Geometry: final body of the model. Coordinates: model frame, mm. Face numbers are marked on the shaded views. A direction names the side the tool comes from. Give positions to 0.01 mm unless a question says otherwise; leave off trailing zeros. Write each loop counter-clockwise with the first axis right and the second up, starting at its lowest first coordinate (ties: lowest second). Pieces come first, ordered by that corner, then holes.
from build123d import *

# Parameters (mm, degrees)
EXTRUDE_1_DEPTH          = 15
SKETCH_2_R               = 5.15
CUT_EXTRUDE_1_DEPTH      = 15
EXTRUDE_3_DEPTH          = 15
SKETCH_5_W               = 5
SKETCH_5_H               = 10
CUT_EXTRUDE_3_DEPTH      = 15
CUT_EXTRUDE_4_DEPTH      = 15
CUT_EXTRUDE_4_DEPTH_BACK = 27
SKETCH_6_R               = 3.25
SKETCH_7_R               = 1.5
CUT_EXTRUDE_5_DEPTH      = 3.5
CUT_EXTRUDE_7_DEPTH      = 15
EXTRUDE_4_REACH          = 135.688
SKETCH_12_R              = 1.75
CUT_EXTRUDE_9_DEPTH      = 50
CUT_EXTRUDE_10_DEPTH     = 3
SKETCH_14_R              = 1.65
CUT_EXTRUDE_11_DEPTH     = 5
SKETCH_15_R              = 5.15
CUT_EXTRUDE_12_DEPTH     = 15
CUT_EXTRUDE_13_DEPTH     = 15
CUT_EXTRUDE_14_DEPTH     = 15
SKETCH_18_W              = 30
SKETCH_18_H              = 15
CUT_EXTRUDE_15_DEPTH     = 15
CUT_EXTRUDE_16_DEPTH     = 135
FILLET_3_R               = 10
FILLET_4_R               = 2
FILLET_5_R               = 5
EXTRUDE_5_DEPTH          = 5
FILLET_6_R               = 1
CUT_EXTRUDE_17_DEPTH     = 0.5
SKETCH_22_R              = 1.65
EXTRUDE_6_DEPTH          = 0.5
SCALE_1_SCALE            = 0.6


with BuildPart() as part:
    # 草图1 → 凸台-拉伸1 (new body)
    with BuildSketch(Plane.XY):
        with BuildLine():
            Line((40, 7.5), (-40, 7.5))
            Line((-40, 7.5), (-40, -7.5))
            Line((-40, -7.5), (39.456922296, -7.5))
            add(Edge.make_bspline(
                [(39.456922296, -7.5), (46.411815441, -13.348879485), (59.483442953, -20.788944656), (71.646457346, -24.94425278), (84, -26.35191574), (96.353542654, -24.94425278), (108.516557047, -20.788944656), (123.382931224, -12.327351589), (132.036036764, -4.43964044)],
                knots=[0.037726639, 0.037726639, 0.037726639, 0.1875, 0.3125, 0.4375, 0.5625, 0.6875, 0.8125, 1, 1, 1], degree=2))
            Line((132.036036764, -4.43964044), (123.963963236, 4.43964044))
            add(Edge.make_bspline(
                [(44.036036764, 4.43964044), (51.882931224, -2.672648411), (64.516557047, -9.836055344), (74.353542654, -13.18074722), (84, -14.27308426), (93.646457346, -13.18074722), (103.483442953, -9.836055344), (116.117068776, -2.672648411), (123.963963236, 4.43964044)],
                knots=[0, 0, 0, 0.1875, 0.3125, 0.4375, 0.5625, 0.6875, 0.8125, 1, 1, 1], degree=2))
            Line((44.036036764, 4.43964044), (40, 7.5))
        make_face()
    extrude(amount=EXTRUDE_1_DEPTH)

    # 草图2 → 切除-拉伸1 (cut)
    with BuildSketch(Plane(origin=(0, 7.5, 0), x_dir=(1, 0, 0), z_dir=(0, 1, 0))):
        with Locations(Location((0, -7.5, 0), (0, 0, 270))):
            Circle(SKETCH_2_R)
    extrude(amount=-CUT_EXTRUDE_1_DEPTH, mode=Mode.SUBTRACT)

    # 草图4 → 凸台-拉伸3 (add)
    with BuildSketch(Plane(origin=(0, 0, 0), x_dir=(-1, 0, 0), z_dir=(0, 0, -1))):
        Polygon((-40, 7.5), (-44.036036764, 7.5), (-44.036036764, 4.43964044), align=None)
    extrude(amount=-EXTRUDE_3_DEPTH)

    # 草图5 → 切除-拉伸3 (cut)
    with BuildSketch(Plane(origin=(0, 0, 0), x_dir=(-1, 0, 0), z_dir=(0, 0, -1))):
        with Locations((-11.65, 2.5)):
            Rectangle(SKETCH_5_W, SKETCH_5_H)
    extrude(amount=-CUT_EXTRUDE_3_DEPTH, mode=Mode.SUBTRACT)

    # 草图6 → 切除-拉伸4 (cut, two sides: drawn at the far end of the back side and taken through both)
    with BuildSketch(Plane(origin=(44.036036764, 0, 0), x_dir=(0, 0, -1), z_dir=(1, 0, 0)).offset(-CUT_EXTRUDE_4_DEPTH_BACK)):
        with Locations(Location((-7.5, 2.5, 0), (0, 0, 143.358054803))):
            Circle(SKETCH_6_R)
    extrude(amount=CUT_EXTRUDE_4_DEPTH + CUT_EXTRUDE_4_DEPTH_BACK, mode=Mode.SUBTRACT)

    # 草图7 → 切除-拉伸5 (cut)
    with BuildSketch(Plane(origin=(9.15, 0, 0), x_dir=(0, 0, -1), z_dir=(1, 0, 0))):
        with Locations((-7.5, 2.5)):
            Circle(SKETCH_7_R)
    extrude(amount=-CUT_EXTRUDE_5_DEPTH, mode=Mode.SUBTRACT)

    # 草图9 → 切除-拉伸7 (cut)
    with BuildSketch(Plane(origin=(0, 0, 0), x_dir=(-1, 0, 0), z_dir=(0, 0, -1))):
        with BuildLine():
            Line((-49, -14.628935139), (-119, -14.628935139))
            add(Edge.make_bspline(
                [(-49, -14.628935139), (-51.259755236, -16.108213622), (-59.483442953, -20.788944656), (-71.646457346, -24.94425278), (-84, -26.35191574), (-96.353542654, -24.94425278), (-108.516557047, -20.788944656), (-116.740244764, -16.108213622), (-119, -14.628935139)],
                knots=[0.139633208, 0.139633208, 0.139633208, 0.1875, 0.3125, 0.4375, 0.5625, 0.6875, 0.8125, 0.860366792, 0.860366792, 0.860366792], degree=2))
        make_face()
    extrude(amount=-CUT_EXTRUDE_7_DEPTH, mode=Mode.SUBTRACT)

    # 凸台-拉伸4: up to this face of the body (flat: up to its plane)
    extrude_4_end = Plane(part.part.faces().sort_by_distance((30.242148565, -2.823725013, 15))[0])
    # 草图10 → 凸台-拉伸4 (add, up to the picked face)
    with BuildSketch(Plane(origin=(0, 0, 0), x_dir=(-1, 0, 0), z_dir=(0, 0, -1)), mode=Mode.PRIVATE) as extrude_4_sk1:
        with BuildLine():
            Line((-114, -3.531559291), (-54, -3.531559291))
            add(Edge.make_bspline(
                [(-54, -3.531559291), (-56.748654683, -5.431567952), (-64.516557047, -9.836055344), (-74.353542654, -13.18074722), (-84, -14.27308426), (-93.646457346, -13.18074722), (-103.483442953, -9.836055344), (-111.251345317, -5.431567952), (-114, -3.531559291)],
                knots=[0.120356468, 0.120356468, 0.120356468, 0.1875, 0.3125, 0.4375, 0.5625, 0.6875, 0.8125, 0.879643532, 0.879643532, 0.879643532], degree=2))
        make_face()
    extrude_4_tool1 = split(extrude(extrude_4_sk1.sketch, amount=-EXTRUDE_4_REACH, mode=Mode.PRIVATE), bisect_by=extrude_4_end, keep=Keep.BOTH, mode=Mode.PRIVATE)
    add(extrude_4_tool1.solids().sort_by(Axis((84, -7.71433, 0), (0, 0, 1)))[0])

    # 草图12 → 切除-拉伸9 (cut)
    with BuildSketch(Plane(origin=(0, -3.531559291, 0), x_dir=(1, 0, 0), z_dir=(0, 1, 0))):
        with Locations(Location((74.000000001, -7.5, 0), (0, 0, 180))):
            Circle(SKETCH_12_R)
        with Locations(Location((104.000000001, -7.5, 0), (0, 0, 180))):
            Circle(SKETCH_12_R)
    extrude(amount=-CUT_EXTRUDE_9_DEPTH, mode=Mode.SUBTRACT)

    # 草图13 → 切除-拉伸10 (cut)
    with BuildSketch(Plane.XZ.offset(14.628935139)):
        Polygon((75.674315782, 4.6), (77.348631563, 7.5), (75.674315782, 10.4), (72.325684221, 10.4), (70.65136844, 7.5), (72.325684221, 4.6), align=None)
        Polygon((105.674315782, 4.6), (107.348631563, 7.5), (105.674315782, 10.4), (102.325684221, 10.4), (100.65136844, 7.5), (102.325684221, 4.6), align=None)
    extrude(amount=-CUT_EXTRUDE_10_DEPTH, mode=Mode.SUBTRACT)

    # 草图14 → 切除-拉伸11 (cut)
    with BuildSketch(Plane(origin=(17.036036764, 0, 0), x_dir=(0, 0, -1), z_dir=(1, 0, 0))):
        with Locations((-7.5, 2.5)):
            Circle(SKETCH_14_R)
    extrude(amount=-CUT_EXTRUDE_11_DEPTH, mode=Mode.SUBTRACT)

    # 草图15 → 切除-拉伸12 (cut)
    with BuildSketch(Plane(origin=(0, 7.5, 0), x_dir=(1, 0, 0), z_dir=(0, 1, 0))):
        with Locations(Location((26.05, -7.5, 0), (0, 0, 270))):
            Circle(SKETCH_15_R)
    extrude(amount=-CUT_EXTRUDE_12_DEPTH, mode=Mode.SUBTRACT)

    # 草图16 → 切除-拉伸13 (cut)
    with BuildSketch(Plane(origin=(0, 0, 0), x_dir=(-1, 0, 0), z_dir=(0, 0, -1))):
        Polygon((-44.036036764, 4.43964044), (-40.036036764, 7.5), (-44.036036764, 7.5), align=None)
    extrude(amount=-CUT_EXTRUDE_13_DEPTH, mode=Mode.SUBTRACT)

    # 草图17 → 切除-拉伸14 (cut)
    with BuildSketch(Plane(origin=(0, 0, 0), x_dir=(-1, 0, 0), z_dir=(0, 0, -1))):
        Polygon((-114, -3.531559291), (-155.45087664, -3.531559291), (-96.986746886, 29.708253825), align=None)
    extrude(amount=-CUT_EXTRUDE_14_DEPTH, mode=Mode.SUBTRACT)

    # 草图18 → 切除-拉伸15 (cut)
    with BuildSketch(Plane(origin=(0, 0, 0), x_dir=(-1, 0, 0), z_dir=(0, 0, -1))):
        with Locations((25, 0)):
            Rectangle(SKETCH_18_W, SKETCH_18_H)
    extrude(amount=-CUT_EXTRUDE_15_DEPTH, mode=Mode.SUBTRACT)

    # 草图19 → 切除-拉伸16 (cut)
    with BuildSketch(Plane.XY.offset(15)):
        Polygon((119, -14.628935139), (127.815134708, -3.531559292), (136.052125617, -3.531559292), align=None)
    extrude(amount=-CUT_EXTRUDE_16_DEPTH, mode=Mode.SUBTRACT)

    # 圆角3
    fillet_3_edges = [part.edges().sort_by_distance(p)[0] for p in [
        (119, -14.628935139, 7.5),
    ]]
    fillet(fillet_3_edges, radius=FILLET_3_R)

    # 圆角4
    fillet_4_edges = [part.edges().sort_by_distance(p)[0] for p in [
        (127.815134708, -3.531559292, 7.5),
    ]]
    fillet(fillet_4_edges, radius=FILLET_4_R)

    # 圆角5
    fillet_5_edges = [part.edges().sort_by_distance(p)[0] for p in [
        (-10, 0, 15),
        (-10, 0, 0),
    ]]
    fillet(fillet_5_edges, radius=FILLET_5_R)

    # 草图20 → 凸台-拉伸5 (add)
    with BuildSketch(Plane(origin=(9.15, 0, 0), x_dir=(0, 0, -1), z_dir=(1, 0, 0))):
        Polygon((-10, -2.5), (-15, -2.5), (-15, 5.5), align=None)
        Polygon((0, 5.5), (-5, -2.5), (0, -2.5), align=None)
    extrude(amount=EXTRUDE_5_DEPTH)

    # 圆角6
    fillet_6_edges = [part.edges().sort_by_distance(p)[0] for p in [
        (11.65, 5.5, 15),
        (11.65, 5.5, 0),
    ]]
    fillet(fillet_6_edges, radius=FILLET_6_R)

    # 草图21 → 切除-拉伸17 (cut)
    with BuildSketch(Plane(origin=(9.15, 0, 0), x_dir=(0, 0, -1), z_dir=(1, 0, 0))):
        with BuildLine():
            Line((-5, -2.5), (-1.847998304, 2.543202714))
            ThreePointArc((-1.847998304, 2.543202714), (-0.724317487, 2.97445252), (0, 2.013203774))
            Line((0, 2.013203774), (0, 7.5))
            Line((0, 7.5), (-15, 7.5))
            Line((-15, 7.5), (-15, 2.013203774))
            ThreePointArc((-15, 2.013203774), (-14.275682513, 2.97445252), (-13.152001696, 2.543202714))
            Line((-13.152001696, 2.543202714), (-10, -2.5))
            Line((-10, -2.5), (-5, -2.5))
        make_face()
    extrude(amount=-CUT_EXTRUDE_17_DEPTH, mode=Mode.SUBTRACT)

    # 草图22 → 凸台-拉伸6 (add)
    with BuildSketch(Plane.ZY.offset(-14.15)):
        with BuildLine():
            Line((0, 7.5), (0, 2.013203774))
            ThreePointArc((0, 2.013203774), (0.724317487, 2.97445252), (1.847998304, 2.543202714))
            Line((1.847998304, 2.543202714), (5, -2.5))
            Line((5, -2.5), (10, -2.5))
            Line((10, -2.5), (13.152001696, 2.543202714))
            ThreePointArc((13.152001696, 2.543202714), (14.275682513, 2.97445252), (15, 2.013203774))
            Line((15, 2.013203774), (15, 7.5))
            Line((15, 7.5), (0, 7.5))
        make_face()
        with Locations(Location((7.5, 2.5, 0), (0, 0, 180))):
            Circle(SKETCH_22_R, mode=Mode.SUBTRACT)
    extrude(amount=EXTRUDE_6_DEPTH)


with BuildPart() as part_1:
    # 缩放比例1: scaled about (0, 0, 0)
    add(part.part.scale(SCALE_1_SCALE))


solid = part_1.part
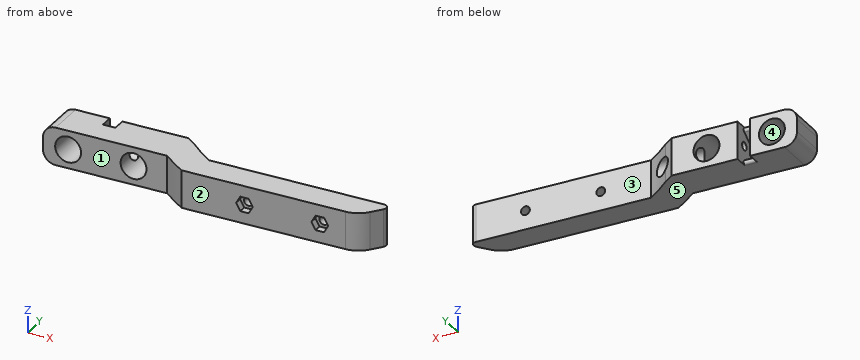
Q1. Section C-C on x = 15.63. Output: boundary loops of the cut face in (y, z).
Filled sheet:
outline: (-4.5, 0) - (4.5, 0) - (4.5, 1.41) - (-4.5, 1.41) - close; (-4.5, 7.59) - (4.5, 7.59) - (4.5, 9) - (-4.5, 9) - close
Q2. Pull-direction query (Z, two-part tool) for the marked faces 3, 4 and 5; classes: released by +Z, released by -Z, zero draft, split by the parting line, or undercut.
Filled sheet:
face 3: zero draft
face 4: undercut
face 5: released by -Z
Q3. Ray query, line 1 along Z through (x, y) = (62.4, -3.75); line 2 along X through (y, z) = (-1.75, 6); line 3 along X through (y, z) = (2.25, 5.75). Return the intervals inside material, ascending.
Filled sheet:
line 1: z = 0 to 3.45, 5.55 to 9
line 2: x = -6 to -2.7, 2.7 to 12.93, 18.33 to 31.87
line 3: x = -6 to -2.83, 2.83 to 5.19, 8.19 to 10.22
Q4. Section B-B on y = -3.25. Output: boundary loops of the cut face in (x, z), plus the area to 3 significant figures.
Filled sheet:
outline: (-6, 3) arc R3 ccw to (-3, 0) - (75.4, 0) - (75.4, 9) - (-3, 9) arc R3 ccw to (-6, 6) - close; hole circle Ø6.18 at (0, 4.5); hole circle Ø6.18 at (15.63, 4.5); hole circle Ø2.1 at (44.4, 4.5); hole circle Ø2.1 at (62.4, 4.5)
area: 662 mm2
Q5. Pin query (flat end, axial travel): P1, Ø4.5, axis at y = 1.5, z = 4.5, coming from the +X side; P2, Ø0.9, axis at x = 63, y = -7.5, coming from the -Z side; P3, Ø1.7, axis at x = 62.4, z = 4.5, coming from the -Y side; P4, Ø0.9, axis at x = 6.5, z = 4, coming from the +Y side. Return the tip coordinate at first contact, or that it passes through.
Filled sheet:
P1: stops at x = 30.51
P2: stops at z = 0
P3: passes through
P4: stops at y = -1.5
Q6. Access query for the marked faces 1 and 2. Directions: +Z, -Z, +X, -X, +Y, -Y. A direction counts if a zero-diameter tool reaches every point of the face in a straight line with its end or side. Return the directions, or none.
Filled sheet:
face 1: +Z, -Z, -X, -Y
face 2: +Z, -Z, +X, -X, -Y
Q7. Section D-D on x = 55. Output: boundary loops of the cut face in (y, z), plus the area to 3 significant figures.
Filled sheet:
outline: (-8.78, 0) - (-2.12, 0) - (-2.12, 9) - (-8.78, 9) - close
area: 59.9 mm2
Q8. Section A-A on x = 44.4. Output: boundary loops of the cut face in (y, z), plus the area to 3 significant figures.
Filled sheet:
outline: (-8.78, 0) - (-2.12, 0) - (-2.12, 3.45) - (-6.98, 3.45) - (-6.98, 2.76) - (-8.78, 2.76) - close; (-8.78, 6.24) - (-6.98, 6.24) - (-6.98, 5.55) - (-2.12, 5.55) - (-2.12, 9) - (-8.78, 9) - close
area: 43.5 mm2
